Read the model definition and answer for the solid it produces. Units are mm, in the model's axes. Face numbers are marked on the shaded views. A direction names the side the tool comes from. Coordinates: 2 decimals unless noted, no trailing zeros. Loops run counter-clockwise (first coordinate to the right, second up) from the corner with the lowest first, then second, coordinate; pieces in that order, holes last.
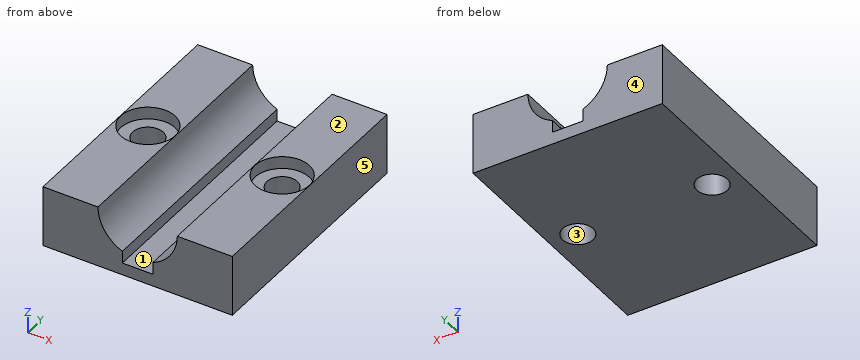
from build123d import *

# Parameters (mm, degrees)
SKETCH1_W           = 31
SKETCH1_H           = 40
BOSS_EXTRUDE1_DEPTH = 10
SKETCH2_R           = 6.5
CUT_EXTRUDE1_DEPTH  = 49.040022953
SKETCH3_R           = 2.5
CUT_EXTRUDE2_DEPTH  = 36.549524257
SKETCH3_4_R         = 4.45
SKETCH3_4_R_2       = 2.5
CUT_EXTRUDE5_DEPTH  = 2
SKETCH4_W           = 5
SKETCH4_H           = 3
CUT_EXTRUDE6_DEPTH  = 49.040022953


with BuildPart() as part:
    # Sketch1 → Boss-Extrude1 (new body)
    with BuildSketch(Plane.XY):
        with Locations((-9.154488543, 3.578059072)):
            Rectangle(SKETCH1_W, SKETCH1_H)
    extrude(amount=BOSS_EXTRUDE1_DEPTH)

    # Sketch2 → Cut-Extrude1 (cut, through all)
    with BuildSketch(Plane(origin=(0, 23.578059072, 0), x_dir=(1, 0, 0), z_dir=(0, 1, 0))):
        with Locations((-9.154488543, -10)):
            Circle(SKETCH2_R)
    extrude(amount=-CUT_EXTRUDE1_DEPTH, mode=Mode.SUBTRACT)

    # Sketch3 → Cut-Extrude2 (cut, through all)
    with BuildSketch(Plane.XY.offset(10)):
        with Locations((-20.154488543, 3.578059072)):
            Circle(SKETCH3_R)
        with Locations((1.845511457, 3.578059072)):
            Circle(SKETCH3_R)
    extrude(amount=-CUT_EXTRUDE2_DEPTH, mode=Mode.SUBTRACT)

    # Sketch3<4> → Cut-Extrude5 (cut)
    # profile 1 of 2: a face of its own
    with BuildSketch(Plane.XY.offset(10)):
        with Locations((-20.154488543, 3.578059072)):
            Circle(SKETCH3_4_R)
        with Locations((-20.154488543, 3.578059072)):
            Circle(SKETCH3_4_R_2, mode=Mode.SUBTRACT)
    # profile 2 of 2: a face of its own
    with BuildSketch(Plane.XY.offset(10)):
        with Locations((1.845511457, 3.578059072)):
            Circle(SKETCH3_4_R)
        with Locations((1.845511457, 3.578059072)):
            Circle(SKETCH3_4_R_2, mode=Mode.SUBTRACT)
    extrude(amount=-CUT_EXTRUDE5_DEPTH, mode=Mode.SUBTRACT)

    # Sketch4 → Cut-Extrude6 (cut, through all)
    with BuildSketch(Plane(origin=(0, 23.578059072, 0), x_dir=(1, 0, 0), z_dir=(0, 1, 0))):
        with Locations((-9.154488543, -3.5)):
            Rectangle(SKETCH4_W, SKETCH4_H)
    extrude(amount=-CUT_EXTRUDE6_DEPTH, mode=Mode.SUBTRACT)


solid = part.part
Item 1: Find the intervals of material crossed by line 1 along X through (y, z) = (5.5, 8.25); line 2 along X through (y, z) = (2, 1.5); line 3 along X through (y, z) = (11.5, 9), in increasing order.
Numbers:
line 1: x = -24.65 to -24.17, -16.14 to -15.41, -2.89 to -2.17, 5.86 to 6.35
line 2: x = -24.65 to -22.09, -18.22 to -0.09, 3.78 to 6.35
line 3: x = -24.65 to -15.58, -2.73 to 6.35
Item 2: Which of the six approach directions +Z, -Z, +X, -X, +Y, -Y give full straight-line access (tool end or side, diameter ignored) to the marked faces 1 and 2?
Numbers:
face 1: +Z, +Y, -Y
face 2: +Z, +X, -X, +Y, -Y
Item 3: A cutting plane is placed at A-A on z = 7. Determine the outline of the cut face in (x, y).
Numbers:
outline: (-24.65, -16.42) - (-14.92, -16.42) - (-14.92, 23.58) - (-24.65, 23.58) - close; (-3.39, -16.42) - (6.35, -16.42) - (6.35, 23.58) - (-3.39, 23.58) - close; hole circle Ø5 at (-20.15, 3.58); hole circle Ø5 at (1.85, 3.58)
Item 4: Determine the mould class of the marked faces 3, 4 and 5 for opening direction X: released by +X, released by -X, zero draft, split by the parting line, or undercut.
Numbers:
face 3: undercut
face 4: zero draft
face 5: released by +X
Item 5: A cutting plane is placed at D-D on z = 1. Determine the outline of the cut face in (x, y).
Numbers:
outline: (-24.65, -16.42) - (6.35, -16.42) - (6.35, 23.58) - (-24.65, 23.58) - close; hole circle Ø5 at (-20.15, 3.58); hole circle Ø5 at (1.85, 3.58)
Item 6: A cutting plane is placed at B-B on y = -11.5. Determine the outline of the cut face in (x, z), then the cut area to 3 significant figures.
Numbers:
outline: (-24.65, 0) - (6.35, 0) - (6.35, 10) - (-2.65, 10) arc R6.5 cw to (-6.65, 4) - (-6.65, 2) - (-11.65, 2) - (-11.65, 4) arc R6.5 cw to (-15.65, 10) - (-24.65, 10) - close
area: 235 mm2
Item 7: Given pin 1 (1.5 mm diameter, centred on x = -9, y = 3, fed in from +Z); pin 2 (8 mm diameter, centred on x = 1.85, y = 3.58, fed in from +Z), each flat-ended and moving along its own axis, determine where each tip first touches the part or whether it passes through.
Numbers:
pin 1: stops at z = 2
pin 2: stops at z = 8
Item 8: A cutting plane is placed at C-C on x = -21.5. Determine the outline of the cut face in (y, z), then the cut area to 3 significant figures.
Numbers:
outline: (-16.42, 0) - (1.47, 0) - (1.47, 8) - (-0.66, 8) - (-0.66, 10) - (-16.42, 10) - close; (5.69, 0) - (23.58, 0) - (23.58, 10) - (7.82, 10) - (7.82, 8) - (5.69, 8) - close
area: 349 mm2
